Design review of the part shown in the three views and the two pictorial views. Dimensions are in mm from the part's minimum x, y and z. A direction names the side the tool comes from. Round coordinates to 2 decimals unless told otherwise and drop trailing zeros. Write each loop counter-clockwise with the first axis right and the second up, starting at its lowest first coordinate (ties: lowest second). Pieces come first, ordered by that corner, then holes. Notation, with made-up numbers: (30, -8.5) -> (62, -8.5) arc R14 cw to (62, -3.5) -> close; hole circle Ø2 at (85, 78.5). An arc over 180 degrees is marked (long way). One line per question, with ' | ' between items. Start each with the question number.
1) Consider section D-D (x = 40). Give the boundary of the cut face in (y, z).
2) Consider section A-A (x = 76.2). Give the boundary of the cut face in (y, z) (3 decimals), then the cut area to 3 significant figures.
3) Consider section C-C (y = 17). Give the boundary of the cut face in (x, z) (3 decimals).
4) For probe 1 along Y at (x, z) = (147.4, 1.15); probe 2 along X at (y, z) = (128.5, 1.55); probe 3 along Z at (x, y) = (36, 67.5), list the stretches that pass through material, from the lowest coordinate up.
5) Consider section B-B (z = 8.7). Give the boundary of the cut face in (x, y) (3 decimals), then the cut area to 3 significant figures.
6) Insertion check: pin 1 Ø2.5 at (x, y) = (5, 128.5) entering from -Z (3 decimals); pin 2 Ø5 at (x, y) = (29, 128.5) entering from +Z; pin 3 Ø5 at (x, y) = (5, 23.9) entering from -Z; pin 4 Ø8 at (y, z) = (39.5, 8) entering from -X. Each pin has a flat end and moves straight along its axis. Give the tip position at first contact, or say it passes through.
7) For the marked faces 1, 2 and 3, list the 3-axis set-ups (+Z, -Z, +X, -X, +Y, -Y) from which the entire face can be reached by the end or side of a thin tool; tool diameter is ignored.
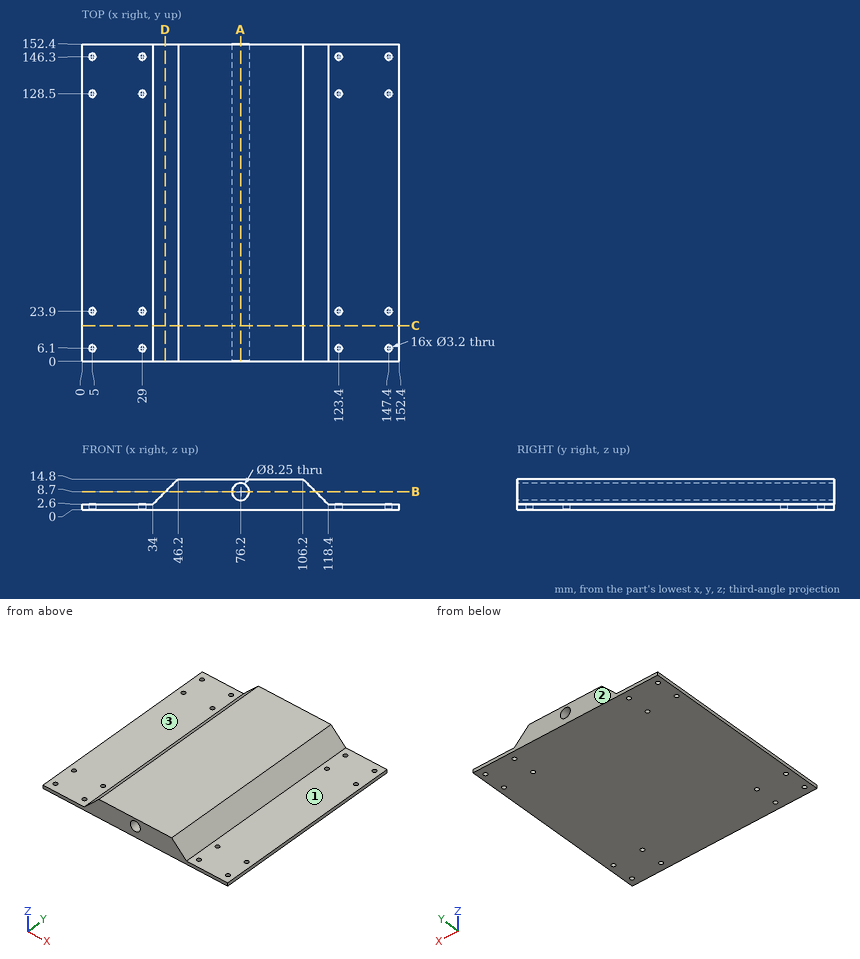
From the geometry:
1) outline: (0, 0) -> (152.4, 0) -> (152.4, 8.6) -> (0, 8.6) -> close
2) outline: (0, 0) -> (152.4, 0) -> (152.4, 4.575) -> (0, 4.575) -> close; (0, 12.825) -> (152.4, 12.825) -> (152.4, 14.8) -> (0, 14.8) -> close | area: 998 mm2
3) outline: (0, 0) -> (152.4, 0) -> (152.4, 2.6) -> (118.4, 2.6) -> (106.2, 14.8) -> (46.2, 14.8) -> (34, 2.6) -> (0, 2.6) -> close; hole circle Ø8.25 at (76.2, 8.7)
4) probe 1: y = 0 to 4.5, 7.7 to 22.3, 25.5 to 126.9, 130.1 to 144.7, 147.9 to 152.4 | probe 2: x = 0 to 3.4, 6.6 to 27.4, 30.6 to 121.8, 125 to 145.8, 149 to 152.4 | probe 3: z = 0 to 4.6
5) outline: (40.1, 0) -> (72.075, 0) -> (72.075, 152.4) -> (40.1, 152.4) -> close; (80.325, 0) -> (112.3, 0) -> (112.3, 152.4) -> (80.325, 152.4) -> close | area: 9,750 mm2
6) pin 1: passes through | pin 2: stops at z = 2.6 | pin 3: stops at z = 0 | pin 4: stops at x = 35.4
7) face 1: +Z, +X, +Y, -Y | face 2: +Z, -Z, +X, -X, +Y | face 3: +Z, -X, +Y, -Y
